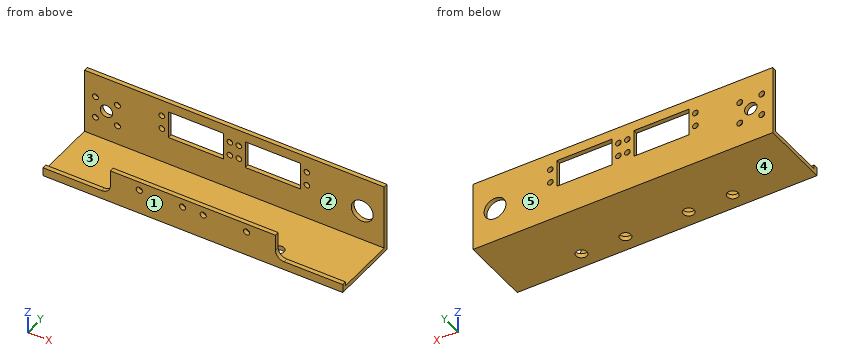
```python
from build123d import *

# Parameters (mm, degrees)
BASE_ANGLE_PROFILE_DEPTH         = 109
SKETCH2_R                        = 2.05
SKETCH2_W                        = 40
SKETCH2_H                        = 20
SERVO_MOUNT_PATTERN_DEPTH        = 3.175
SKETCH3_R                        = 4.5
SKETCH3_R_2                      = 2.15
LEAD_SCREW_NUT_PATTERN_DEPTH     = 3.175
SKETCH4_R                        = 7.9375
SUPPORT_SHAFT_PASS_THROUGH_DEPTH = 3.175
CHANNEL_BOTTOM_CUT_DEPTH         = 10
SKETCH7_R                        = 4
CUT_EXTRUDE5_DEPTH               = 4.175
SKETCH8_R                        = 2.25
CUT_EXTRUDE6_DEPTH               = 3.175
FILLET1_R                        = 6.35
BODY_MOVE_COPY1_ANGLE            = 180


with BuildPart() as part:
    # Sketch1 → Base Angle Profile (new body, symmetric)
    with BuildSketch(Plane(origin=(0, 0, 0), x_dir=(0, 0, -1), z_dir=(1, 0, 0))):
        Polygon((0, 0), (50.8, 0), (50.8, -3.175), (3.175, -3.175), (3.175, -47.625), (50.8, -47.625), (50.8, -50.8), (0, -50.8), align=None)
    extrude(amount=BASE_ANGLE_PROFILE_DEPTH, both=True)

    # Sketch2 → Servo Mount Pattern (cut)
    with BuildSketch(Plane(origin=(0, 0, 0), x_dir=(1, 0, 0), z_dir=(0, 1, 0))):
        with Locations((-52.75, 38.8)):
            Circle(SKETCH2_R)
        with Locations((-52.75, 28.8)):
            Circle(SKETCH2_R)
        with Locations((-3.25, 38.8)):
            Circle(SKETCH2_R)
        with Locations((-3.25, 28.8)):
            Circle(SKETCH2_R)
        with Locations((3.25, 28.8)):
            Circle(SKETCH2_R)
        with Locations((3.25, 38.8)):
            Circle(SKETCH2_R)
        with Locations((52.75, 38.8)):
            Circle(SKETCH2_R)
        with Locations((52.75, 28.8)):
            Circle(SKETCH2_R)
        with Locations((-28, 33.8)):
            Rectangle(SKETCH2_W, SKETCH2_H)
        with Locations((28, 33.8)):
            Rectangle(SKETCH2_W, SKETCH2_H)
    extrude(amount=-SERVO_MOUNT_PATTERN_DEPTH, mode=Mode.SUBTRACT)

    # Sketch3 → Lead Screw Nut Pattern (cut)
    with BuildSketch(Plane(origin=(0, 0, 0), x_dir=(1, 0, 0), z_dir=(0, 1, 0))):
        with Locations((93, 25.4)):
            Circle(SKETCH3_R)
        with Locations((101, 33.4)):
            Circle(SKETCH3_R_2)
        with Locations((85, 33.4)):
            Circle(SKETCH3_R_2)
        with Locations((85, 17.4)):
            Circle(SKETCH3_R_2)
        with Locations((101, 17.4)):
            Circle(SKETCH3_R_2)
    extrude(amount=-LEAD_SCREW_NUT_PATTERN_DEPTH, mode=Mode.SUBTRACT)

    # Sketch4 → Support Shaft Pass Through (cut)
    with BuildSketch(Plane(origin=(0, 0, 0), x_dir=(1, 0, 0), z_dir=(0, 1, 0))):
        with Locations((-93, 25.4)):
            Circle(SKETCH4_R)
    extrude(amount=-SUPPORT_SHAFT_PASS_THROUGH_DEPTH, mode=Mode.SUBTRACT)

    # Sketch5 → Channel Bottom Cut (cut)
    with BuildSketch(Plane.XZ.offset(50.8)):
        Polygon((-109, -6.175), (-60, -6.175), (-60, -24.205), (60, -24.205), (60, -6.175), (109, -6.175), (109, -50.8), (-109, -50.8), align=None)
    extrude(amount=-CHANNEL_BOTTOM_CUT_DEPTH, mode=Mode.SUBTRACT)

    # Sketch7 → Cut-Extrude5 (cut, through all)
    with BuildSketch(Plane(origin=(0, 0, -3.175), x_dir=(-1, 0, 0), z_dir=(0, 0, -1))):
        with Locations((-55, -39.295)):
            Circle(SKETCH7_R)
        with Locations((-23, -39.295)):
            Circle(SKETCH7_R)
        with Locations((23, -39.295)):
            Circle(SKETCH7_R)
        with Locations((55, -39.295)):
            Circle(SKETCH7_R)
    extrude(amount=-CUT_EXTRUDE5_DEPTH, mode=Mode.SUBTRACT)

    # Sketch8 → Cut-Extrude6 (cut)
    with BuildSketch(Plane(origin=(0, -50.8, 0), x_dir=(-1, 0, 0), z_dir=(0, -1, 0))):
        with Locations((39, 17.955)):
            Circle(SKETCH8_R)
        with Locations((7.5, 17.955)):
            Circle(SKETCH8_R)
        with Locations((-7.5, 17.955)):
            Circle(SKETCH8_R)
        with Locations((-39, 17.955)):
            Circle(SKETCH8_R)
    extrude(amount=-CUT_EXTRUDE6_DEPTH, mode=Mode.SUBTRACT)

    # Fillet1
    fillet1_edges = [part.edges().sort_by_distance(p)[0] for p in [
        (-60, -49.2125, -6.175),
        (60, -49.2125, -6.175),
    ]]
    fillet(fillet1_edges, radius=FILLET1_R)


with BuildPart() as part_1:
    # Body-Move/Copy1: moved
    add(part.part.rotate(Axis((0, 0, -25.4), (0, 1, 0)), BODY_MOVE_COPY1_ANGLE))


solid = part_1.part
```
Work out the finished part from the listing and answer in its coordinate system (mm). Face numbers are marked on the shaded views. A direction names the side the tool comes from. Give positions to 0.01 mm unless a question says otherwise; leave off trailing zeros. Loops run counter-clockwise (first coordinate to the right, second up) from the corner with the lowest first, then second, coordinate; pieces in that order, holes last. Notation, with made-up numbers: (-37, 65.5) -> (-28, 65.5) arc R6 cw to (-28, 69.5) -> close; hole circle Ø1 at (15, -28). An arc over 180 degrees is marked (long way). Put each result on its own line as item: value. Start each with the question number.
Item 1: The mould has two halves that part along Y. Classify the marked faces 3, 4 and 5: released by +Y, released by -Y, zero draft, split by the parting line, or undercut.
Item 2: The part is cut by section B-B (x = -33.5). Give the vertices of the cut face in (y, z) (3 decimals).
Item 3: The part is cut by section D-D (y = -12.5). Give the vertices of the cut face in (x, z) (3 decimals).
Item 4: Find the intervals of material crossed by L1, parallel to Y at x = 11, z = -31 (3 decimals); L2, parallel to Z at x = 39, y = -48.55 (3 decimals); L3, parallel to Z at x = -85, y = -9.5 (3 decimals), in increasing order. Write a range as [from, to].
Item 5: The part is cut by section C-C (x = 23). Give the vertices of the cut face in (y, z) (3 decimals).
Item 6: Which of the six approach directions +Z, -Z, +X, -X, +Y, -Y give full straight-line access (tool end or side, diameter ignored) to the marked faces 1 and 2?
Item 7: The part is cut by section A-A (x = -101). Give the vertices of the cut face in (y, z) (3 decimals), then the cut area to 3 significant figures.
Item 8: Each of these flat-tipped pins is pushed along its axis until it touches: P1, Ø1, axis at x = -29.5, y = -49.5, coming from the +Z side (3 decimals); P2, Ø3.5, axis at x = 39, z = -32.845, coming from the -Y side (3 decimals); P3, Ø3, axis at x = -10.5, z = -21.5, coming from the -Y side; P4, Ø2.5, axis at y = -49.5, z = -31.5, coming from the +X side. Where does it stop, or does it pass through?
Answers below:
1. face 3: undercut
1. face 4: zero draft
1. face 5: released by +Y
2. outline: (-50.8, -50.8) -> (0, -50.8) -> (0, -27) -> (-3.175, -27) -> (-3.175, -47.625) -> (-47.625, -47.625) -> (-47.625, -26.595) -> (-50.8, -26.595) -> close; (-3.175, -7) -> (0, -7) -> (0, 0) -> (-3.175, 0) -> close
3. outline: (-109, -50.8) -> (109, -50.8) -> (109, -47.625) -> (-109, -47.625) -> close
4. L1: [-50.8, -47.625], [-3.175, 0]
4. L2: [-50.8, -35.095], [-30.595, -26.595]
4. L3: [-50.8, -47.625]
5. outline: (-50.8, -50.8) -> (-43.295, -50.8) -> (-43.295, -47.625) -> (-47.625, -47.625) -> (-47.625, -26.595) -> (-50.8, -26.595) -> close; (-35.295, -50.8) -> (0, -50.8) -> (0, -27) -> (-3.175, -27) -> (-3.175, -47.625) -> (-35.295, -47.625) -> close; (-3.175, -7) -> (0, -7) -> (0, 0) -> (-3.175, 0) -> close
6. face 1: +Z, -Z, +X, -X, -Y
6. face 2: +Z, +X, -X
7. outline: (-50.8, -50.8) -> (0, -50.8) -> (0, -35.55) -> (-3.175, -35.55) -> (-3.175, -47.625) -> (-47.625, -47.625) -> (-47.625, -44.625) -> (-50.8, -44.625) -> close; (-3.175, -31.25) -> (0, -31.25) -> (0, -19.55) -> (-3.175, -19.55) -> close; (-3.175, -15.25) -> (0, -15.25) -> (0, 0) -> (-3.175, 0) -> close
7. area: 295 mm2
8. P1: z = -26.595
8. P2: y = -3.175
8. P3: through
8. P4: x = 60
